```python
from build123d import *

# Parameters (mm, degrees)
F2_DEPTH = 50.8
F4_DEPTH = 88.9
F5_R     = 50.8
F6_R     = 12.7
F7_DEPTH = 25.4


with BuildPart() as f2:
    # F0 (on Front) → F2 (new body, symmetric)
    with BuildSketch(Plane.XZ):
        with BuildLine():
            Line((-76.2, 0), (0, 0))
            Line((0, 0), (76.2, 0))
            ThreePointArc((76.2, 0), (90.5141334361, 22.8530864989), (117.3231151597, 19.948525))
            Line((117.3231151597, 19.948525), (211.6618061177, 139.639675))
            ThreePointArc((211.6618061177, 139.639675), (203.4161012645, 167.9938925468), (227.564983392, 184.9875617564))
            Line((227.564983392, 184.9875617564), (0, 186.6008240309))
            Line((0, 186.6008240309), (-227.564983392, 184.9875617564))
            ThreePointArc((-227.564983392, 184.9875617564), (-209.4881838332, 177.6122613863), (-201.9849212774, 159.5882))
            ThreePointArc((-201.9849212774, 159.5882), (-204.5318347785, 148.5023334361), (-211.6618061177, 139.639675))
            Line((-211.6618061177, 139.639675), (-117.3231151597, 19.948525))
            ThreePointArc((-117.3231151597, 19.948525), (-90.5141334361, 22.8530864989), (-76.2, 0))
        make_face()
        with BuildLine():
            ThreePointArc((-227.564983392, 184.9875617564), (-251.3537412903, 151.1825074532), (-211.6618061177, 139.639675))
            ThreePointArc((-211.6618061177, 139.639675), (-204.5318347785, 148.5023334361), (-201.9849212774, 159.5882))
            ThreePointArc((-201.9849212774, 159.5882), (-209.4881838332, 177.6122613863), (-227.564983392, 184.9875617564))
        make_face()
        with BuildLine():
            ThreePointArc((-214.6849212774, 159.5882), (-215.9583780279, 154.0452667181), (-219.5233636976, 149.6139375))
            ThreePointArc((-219.5233636976, 149.6139375), (-238.8114645269, 165.1311332819), (-214.6849212774, 159.5882))
        make_face(mode=Mode.SUBTRACT)
        with BuildLine():
            ThreePointArc((-117.3231151597, 19.948525), (-112.6858665639, -22.8530864989), (-76.2, 0))
            Line((-76.2, 0), (-88.9, 0))
            ThreePointArc((-88.9, 0), (-107.1429332819, -11.4265432495), (-109.4615575798, 9.9742625))
            Line((-109.4615575798, 9.9742625), (-117.3231151597, 19.948525))
        make_face()
        with BuildLine():
            Line((88.9, 0), (76.2, 0))
            ThreePointArc((76.2, 0), (101.6, -25.4), (127, 0))
            ThreePointArc((127, 0), (124.4530864989, 11.0858665639), (117.3231151597, 19.948525))
            Line((117.3231151597, 19.948525), (109.4615575798, 9.9742625))
            ThreePointArc((109.4615575798, 9.9742625), (113.0265432495, 5.5429332819), (114.3, 0))
            ThreePointArc((114.3, 0), (101.6, -12.7), (88.9, 0))
        make_face()
        with BuildLine():
            ThreePointArc((117.3231151597, 19.948525), (90.5141334361, 22.8530864989), (76.2, 0))
            Line((76.2, 0), (88.9, 0))
            ThreePointArc((88.9, 0), (96.0570667181, 11.4265432495), (109.4615575798, 9.9742625))
            Line((109.4615575798, 9.9742625), (117.3231151597, 19.948525))
        make_face()
        with BuildLine():
            Line((-88.9, 0), (-76.2, 0))
            ThreePointArc((-76.2, 0), (-90.5141334361, 22.8530864989), (-117.3231151597, 19.948525))
            Line((-117.3231151597, 19.948525), (-109.4615575798, 9.9742625))
            ThreePointArc((-109.4615575798, 9.9742625), (-96.0570667181, 11.4265432495), (-88.9, 0))
        make_face()
        with BuildLine():
            ThreePointArc((227.564983392, 184.9875617564), (203.4161012645, 167.9938925468), (211.6618061177, 139.639675))
            ThreePointArc((211.6618061177, 139.639675), (238.4707878413, 136.7351135011), (252.7849212774, 159.5882))
            ThreePointArc((252.7849212774, 159.5882), (245.4089826636, 177.4849374441), (227.564983392, 184.9875617564))
        make_face()
        with BuildLine():
            ThreePointArc((240.0849212774, 159.5882), (232.9278545593, 148.1616567505), (219.5233636976, 149.6139375))
            ThreePointArc((219.5233636976, 149.6139375), (221.8419879955, 171.0147432495), (240.0849212774, 159.5882))
        make_face(mode=Mode.SUBTRACT)
    extrude(amount=F2_DEPTH, both=True)

    # F3 (on face) → F4 (cut)
    with BuildSketch(Plane(origin=(0, 50.8, 0), x_dir=(-1, 0, 0), z_dir=(0, 1, 0))):
        Polygon((0, 186.6008240309), (-166.8902328226, 185.4176994896), (-60.3365621927, 50.2289318176), (60.3365621927, 50.2289318176), (166.8902328226, 185.4176994896), align=None)
    extrude(amount=-F4_DEPTH, mode=Mode.SUBTRACT)

    # F5
    f5_edges = [f2.edges().sort_by_distance(p)[0] for p in [
        (166.890233, 6.35, 185.417699),
        (-166.890233, 6.35, 185.417699),
        (-60.336562, 6.35, 50.228932),
        (60.336562, 6.35, 50.228932),
    ]]
    fillet(f5_edges, radius=F5_R)

    # F6 (on face) → F7 (cut, symmetric)
    with BuildSketch(Plane.XZ):
        with BuildLine():
            ThreePointArc((206.9448715698, 133.6551175), (241.7965478104, 129.8791875514), (260.4049212774, 159.5882))
            ThreePointArc((260.4049212774, 159.5882), (241.5199905801, 189.4297853434), (206.4666889451, 185.1371325822))
            Line((206.4666889451, 185.1371325822), (227.564983392, 184.9875617564))
            ThreePointArc((227.564983392, 184.9875617564), (203.4161012645, 167.9938925468), (211.6618061177, 139.639675))
            Line((211.6618061177, 139.639675), (206.9448715698, 133.6551175))
        make_face()
        with Locations((227.3849212774, 159.5882)):
            Circle(F6_R, mode=Mode.SUBTRACT)
        with BuildLine():
            ThreePointArc((134.62, 0), (131.3090124486, 14.411626533), (122.0400497076, 25.9330825))
            Line((122.0400497076, 25.9330825), (117.3231151597, 19.948525))
            ThreePointArc((117.3231151597, 19.948525), (90.5141334361, 22.8530864989), (76.2, 0))
            Line((76.2, 0), (68.58, 0))
            ThreePointArc((68.58, 0), (101.6, -33.02), (134.62, 0))
        make_face()
        with Locations((101.6, 0)):
            Circle(F6_R, mode=Mode.SUBTRACT)
        with BuildLine():
            Line((-117.3231151597, 19.948525), (-122.0400497076, 25.9330825))
            ThreePointArc((-122.0400497076, 25.9330825), (-116.011626533, -29.7090124486), (-68.58, 0))
            Line((-68.58, 0), (-76.2, 0))
            ThreePointArc((-76.2, 0), (-90.5141334361, 22.8530864989), (-117.3231151597, 19.948525))
        make_face()
        with Locations((-101.6, 0)):
            Circle(F6_R, mode=Mode.SUBTRACT)
        with BuildLine():
            Line((-227.564983392, 184.9875617564), (-206.4666889451, 185.1371325822))
            ThreePointArc((-206.4666889451, 185.1371325822), (-260.403496997, 159.8948878633), (-206.9448715698, 133.6551175))
            Line((-206.9448715698, 133.6551175), (-211.6618061177, 139.639675))
            ThreePointArc((-211.6618061177, 139.639675), (-204.5318347785, 148.5023334361), (-201.9849212774, 159.5882))
            ThreePointArc((-201.9849212774, 159.5882), (-209.4881838332, 177.6122613863), (-227.564983392, 184.9875617564))
        make_face()
        with Locations((-227.3849212774, 159.5882)):
            Circle(F6_R, mode=Mode.SUBTRACT)
    extrude(amount=F7_DEPTH, both=True, mode=Mode.SUBTRACT)


solid = f2.part
```
Verification items for the finished model (mm, model axes). A direction names the side the tool comes from. Coordinates: 2 decimals unless noted, no trailing zeros. Write each loop counter-clockwise with the first axis right and the second up, starting at its lowest first coordinate (ties: lowest second). Pieces come first, ordered by that corner, then holes. Notation, with made-up numbers: M 32.25,-40 L 51.25,-40 A10 cw 51.25,-29 Z; hole C 1,82 d10. An arc over 180 degrees is marked long. Answer as a JSON object with one key per item and string values. Group by question number.
(1) Cross-section at C-C, the plane y = -4. Record the cut outline in (x, z).
(2) Cross-section at D-D, the plane z = 81. Record the cut outline in (x, y).
(3) Gauge pin test, flat ends, axial feed: pin 1 (1 mm diameter, centred on y = -31, z = 66.5, fed in from +X); pin 2 (2 mm diameter, centred on x = -24, y = 36, fed in from +Z); pin 3 (8 mm diameter, centred on y = -2, z = 108, fed in from -X). Record the tip position at first contact, or that the pin passes through.
(4) Tool access check on faces 1 (the face through (57.576, 5.728, 55.183)), 2 (the face through (90.874, 0.356, 23.024)), 3 (the face through (-20, 50.8, 41)), 4 (the face through (-113.33, 37.92, -22.53)), 5 (the face through (216, 25.4, 166)). Record the directions out of +Z, -Z, +X, -X, +Y, -Y that give a thin tool (end or side, any length) a straight path to the whole face; none if there is none.
(5) Material ranges on line 1 (Z direction, x = -226, y = 30.5); line 2 (X direction, y = -42.5, z = 148.5); line 3 (Y direction, x = -82.5, z = 81.5), recorded low to high.
(6) Release check for a two-part mould opening along Y. For faces 6 (the face through (251.122, -38.278, 150.548)), 7 (the face through (3, -38.1, 135)), 8 (the face through (-90.2, 0.4, 22.7)) record: +Y half, -Y half, draft (parallel to the pull), parting line (faces both ways), or undercut.
(7) Cross-section at B-B, the plane y = 34.5. Record the cut outline in (x, z), and give its area (3 significant figures).
(8) Cross-section at A-A, the plane x = -101.6. Record the cut outline in (y, z), and give its area (3 significant figures).
Reply:
{
 "1": {"outline": "M -227.56,184.99 A25.4 cw -211.66,139.64 L -117.32,19.95 A25.4 cw -76.2,0 L 76.2,0 A25.4 cw 117.32,19.95 L 211.66,139.64 A25.4 cw 227.56,184.99 L 191.76,185.24 A50.8 ccw 151.5,165.89 L 75.59,69.58 A50.8 cw 35.69,50.23 L -35.69,50.23 A50.8 cw -75.59,69.58 L -151.5,165.89 A50.8 ccw -191.76,185.24 Z"},
 "2": {"outline": "M -165.44,-50.8 L 165.44,-50.8 L 165.44,50.8 L 84.59,50.8 L 84.59,-38.1 L -84.59,-38.1 L -84.59,50.8 L -165.44,50.8 Z"},
 "3": {"pin 1": "x = 154.41", "pin 2": "z = 50.23", "pin 3": "x = -189.88"},
 "4": {"face 1": "+Z, +Y", "face 2": "-Z", "face 3": "+Z, -Z, +X, -X, +Y", "face 4": "+Y, -Y", "face 5": "+X"},
 "5": {"line 1": "134.23 to 146.96, 172.21 to 185", "line 2": "-250.24 to -233.58, -221.19 to 221.19, 233.58 to 250.24", "line 3": "-50.8 to -38.1"},
 "6": {"face 6": "draft", "face 7": "+Y half", "face 8": "undercut"},
 "7": {"outline": "M -227.56,184.99 A25.4 ccw long -211.66,139.64 L -117.32,19.95 A25.4 ccw long -76.2,0 L 76.2,0 A25.4 ccw long 117.32,19.95 L 211.66,139.64 A25.4 ccw long 227.56,184.99 L 191.76,185.24 A50.8 ccw 151.5,165.89 L 75.59,69.58 A50.8 cw 35.69,50.23 L -35.69,50.23 A50.8 cw -75.59,69.58 L -151.5,165.89 A50.8 ccw -191.76,185.24 Z; hole C -227.38,159.59 d25.4; hole C -101.6,0 d25.4; hole C 101.6,0 d25.4; hole C 227.38,159.59 d25.4", "area": "36,500 mm²"},
 "8": {"outline": "M -50.8,-25.4 L -25.4,-25.4 L -25.4,-12.7 L -50.8,-12.7 Z; M -50.8,12.7 L -25.4,12.7 L -25.4,25.4 L 25.4,25.4 L 25.4,12.7 L 50.8,12.7 L 50.8,102.58 L -38.1,102.58 L -38.1,185.88 L -50.8,185.88 Z; M 25.4,-25.4 L 50.8,-25.4 L 50.8,-12.7 L 25.4,-12.7 Z", "area": "10,200 mm²"}
}
